Model file for the job. Use its own axes, mm. Round coordinates to 2 decimals unless told otherwise and drop trailing zeros. Loops run counter-clockwise (first coordinate to the right, second up) from the corner with the lowest first, then second, coordinate; pieces in that order, holes last. Notation, with made-up numbers: M 26.25,-12 L 70.25,-12 A11 ccw 70.25,3 Z; hole C 85,-37.5 d3. An arc over 180 degrees is marked long. Use a Markdown table: item, result. Add a question column.
Q1. Probe line 1 (Y direction, x = 120, z = -0.55); line 2 (X direction, y = -75, z = -0.7); line 3 (Y direction, x = -43.5, z = -0.85). List the from-to ranges inside material, lowest first. Write a range as from..to.
Q2. Cut at B-B (z = -0.8). Give the cut face in (x, y).
Q3. Cut at C-C (x = -44.5). Give the cut face in (y, z).
Q4. Cut at A-A (y = -71). Give the cut face in (x, z), plus the area to 3 significant figures.
from build123d import *

# Parameters (mm, degrees)
T_LE_DE_BASE_PLI_E1_DEPTH = 1
ESQUISSE6_R               = 1.5
ESQUISSE6_W               = 18.5
ESQUISSE6_H               = 30.5
ENL_V_MAT_EXTRU_1_DEPTH   = 1
CONG_1_R                  = 3


# Sheet-metal steps are written as plain solids
with BuildPart() as part:
    # Esquisse1 → Tôle de base pliée1 (new body)
    with BuildSketch(Plane.XY):
        Polygon((47.5, -82), (129, -82), (129, 0), (-129, 0), (-129, -82), (-47.5, -82), (-47.5, -65.5), (47.5, -65.5), align=None)
    extrude(amount=-T_LE_DE_BASE_PLI_E1_DEPTH)

    # Esquisse6 → Enlèv. mat.-Extru.1 (cut)
    with BuildSketch(Plane.XY):
        with Locations((-120, -20)):
            Circle(ESQUISSE6_R)
        with Locations(Location((120, -20, 0), (0, 0, 180))):
            Circle(ESQUISSE6_R)
        with Locations((-119.75, -49.75)):
            Rectangle(ESQUISSE6_W, ESQUISSE6_H)
        with Locations((119.75, -49.75)):
            Rectangle(ESQUISSE6_W, ESQUISSE6_H)
    extrude(amount=-ENL_V_MAT_EXTRU_1_DEPTH, mode=Mode.SUBTRACT)

    # Congé1
    cong_1_edges = [part.edges().sort_by_distance(p)[0] for p in [
        (110.5, -65, -0.5),
        (110.5, -34.5, -0.5),
        (-110.5, -34.5, -0.5),
        (-110.5, -65, -0.5),
    ]]
    fillet(cong_1_edges, radius=CONG_1_R)


solid = part.part
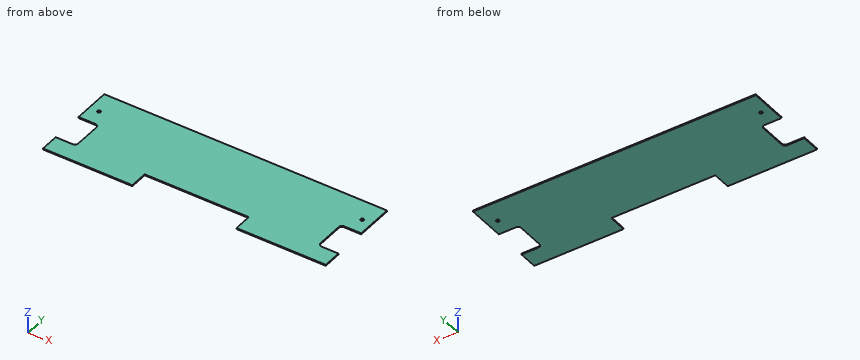
Checked values:
| question | item | result |
|---|---|---|
| 1 | line 1 | y = -82..-65, -34.5..-21.5, -18.5..0 |
| 1 | line 2 | x = -129..-47.5, 47.5..129 |
| 1 | line 3 | y = -65.5..0 |
| 2 | outline | M -129,-82 L -47.5,-82 L -47.5,-65.5 L 47.5,-65.5 L 47.5,-82 L 129,-82 L 129,-65 L 113.5,-65 A3 cw 110.5,-62 L 110.5,-37.5 A3 cw 113.5,-34.5 L 129,-34.5 L 129,0 L -129,0 L -129,-34.5 L -113.5,-34.5 A3 cw -110.5,-37.5 L -110.5,-62 A3 cw -113.5,-65 L -129,-65 Z; hole C -120,-20 d3; hole C 120,-20 d3 |
| 3 | outline | M -65.5,-1 L 0,-1 L 0,0 L -65.5,0 Z |
| 4 | outline | M -129,-1 L -47.5,-1 L -47.5,0 L -129,0 Z; M 47.5,-1 L 129,-1 L 129,0 L 47.5,0 Z |
| 4 | area | 163 mm^2 |
